```python
from build123d import *

# Parameters (mm, degrees)
EXTRUDE_1_DEPTH     = 80
SKETCH_3_R          = 17.5
EXTRUDE_2_DEPTH     = 10
EXTRUDE_START       = 10
SKETCH_4_R          = 17.5
EXTRUDE_3_DEPTH     = 10
SKETCH_6_R          = 9.5
CUT_EXTRUDE_3_DEPTH = 6
CUT_EXTRUDE_START   = -6
SKETCH_7_R          = 9.5
CUT_EXTRUDE_4_DEPTH = 6
SKETCH_8_R          = 6.5
CUT_EXTRUDE_5_DEPTH = 100
SKETCH_11_R         = 14.5
CUT_EXTRUDE_8_DEPTH = 3
SKETCH_13_R         = 17.5
EXTRUDE_5_DEPTH     = 10


with BuildPart() as part:
    # 草图1 → 凸台-拉伸1 (new body)
    with BuildSketch(Plane.XY):
        Polygon((-20, 18), (-18, 20), (17.735809733, 20), (20, 18), (20, -17.735809733), (17.735809733, -20), (-18, -20), (-20, -18), align=None)
    extrude(amount=EXTRUDE_1_DEPTH)

    # 草图3 → 凸台-拉伸2 (add)
    with BuildSketch(Plane.XY.offset(80)):
        Circle(SKETCH_3_R)
    extrude(amount=EXTRUDE_2_DEPTH)

    # 草图4 → 凸台-拉伸3 (add)
    with BuildSketch(Plane(origin=(0, 0, 0), x_dir=(-1, 0, 0), z_dir=(0, 0, -1)).offset(EXTRUDE_START)):
        with Locations(Location((0, 0, 0), (0, 0, 180))):
            Circle(SKETCH_4_R)
    extrude(amount=-EXTRUDE_3_DEPTH)

    # 草图6 → 切除-拉伸3 (cut)
    with BuildSketch(Plane(origin=(0, 0, -10), x_dir=(-1, 0, 0), z_dir=(0, 0, -1))):
        Circle(SKETCH_6_R)
    extrude(amount=-CUT_EXTRUDE_3_DEPTH, mode=Mode.SUBTRACT)

    # 草图7 → 切除-拉伸4 (cut)
    with BuildSketch(Plane.XY.offset(90).offset(CUT_EXTRUDE_START)):
        with Locations(Location((0, 0, 0), (0, 0, 180))):
            Circle(SKETCH_7_R)
    extrude(amount=CUT_EXTRUDE_4_DEPTH, mode=Mode.SUBTRACT)

    # 草图8 → 切除-拉伸5 (cut)
    with BuildSketch(Plane(origin=(0, 0, -10), x_dir=(-1, 0, 0), z_dir=(0, 0, -1))):
        Circle(SKETCH_8_R)
    extrude(amount=-CUT_EXTRUDE_5_DEPTH, mode=Mode.SUBTRACT)

    # 草图11 → 切除-拉伸8 (cut)
    with BuildSketch(Plane.XY.offset(61.11)):
        Polygon((17.735809733, -20), (-18, -20), (-20, -18), (-20, 18), (-18, 20), (17.735809733, 20), (20, 18), (20, -17.735809733), align=None)
        Circle(SKETCH_11_R, mode=Mode.SUBTRACT)
    extrude(amount=-CUT_EXTRUDE_8_DEPTH, mode=Mode.SUBTRACT)

    # 草图13 → 凸台-拉伸5 (add)
    with BuildSketch(Plane.XY.offset(80)):
        Polygon((-20, 18), (-20, -18), (-18, -20), (17.735809733, -20), (20, -17.735809733), (20, 18), (17.735809733, 20), (-18, 20), align=None)
        with Locations(Location((0, 0, 0), (0, 0, 180))):
            Circle(SKETCH_13_R, mode=Mode.SUBTRACT)
    extrude(amount=EXTRUDE_5_DEPTH)


solid = part.part
```
Input: part model. Units: mm. Frame: model coordinates. A direction names the side the tool comes from. Give positions to 0.01 mm unless a question says otherwise; leave off trailing zeros. Order: outer loops, then holes, each group sorted by start corner. A loop starts at its lowest first (then second) coordinate and runs counter-clockwise, first axis right, second up. Notation, with made-up numbers: M -11.5,74.25 L 20.5,74.25 A13 cw 20.5,83.25 Z; hole C -33.5,-10 d10. An arc over 180 degrees is marked long. Return JSON: item names as keys, results as strings.
1) Line query: L1, parallel to Y at x = 0, z = -7.45; L2, parallel to Z at x = -7, y = 13; L3, parallel to Z at x = 17, y = -16.5. Output: solid intervals per line, ascending. Write a range as [from, to].
Taken from the geometry:
{"L1": "y = [-17.5, -9.5], [9.5, 17.5]", "L2": "z = [-10, 58.11], [61.11, 90]", "L3": "z = [0, 58.11], [61.11, 90]"}
2) Section query C-C on z = 41.5. Output: boundary loops of the cut face in (x, y), and give its area (3 significant figures).
Taken from the geometry:
{"outline": "M -20,-18 L -18,-20 L 17.74,-20 L 20,-17.74 L 20,18 L 17.74,20 L -18,20 L -20,18 Z; hole C 0,0 d13", "area": "1,460 mm2"}
3) Section query D-D on x = -16.5. Output: boundary loops of the cut face in (y, z).
Taken from the geometry:
{"outline": "M -20,0 L -5.83,0 L -5.83,-10 L 5.83,-10 L 5.83,0 L 20,0 L 20,58.11 L -20,58.11 Z; M -20,61.11 L 20,61.11 L 20,90 L -20,90 Z"}
4) Contact query for a flat-ended pin moving along its axis: pin 1 (17 mm diameter, centred on x = 0, y = 0, fed in from +Z). Output: stop coordinate, or through.
Taken from the geometry:
{"pin 1": "stops at z = 84"}
5) Section query A-A on x = 0. Output: boundary loops of the cut face in (y, z).
Taken from the geometry:
{"outline": "M -20,0 L -17.5,0 L -17.5,-10 L -9.5,-10 L -9.5,-4 L -6.5,-4 L -6.5,84 L -9.5,84 L -9.5,90 L -20,90 L -20,61.11 L -14.5,61.11 L -14.5,58.11 L -20,58.11 Z; M 6.5,-4 L 9.5,-4 L 9.5,-10 L 17.5,-10 L 17.5,0 L 20,0 L 20,58.11 L 14.5,58.11 L 14.5,61.11 L 20,61.11 L 20,90 L 9.5,90 L 9.5,84 L 6.5,84 Z"}
6) Mould query, pull axis X, two halves, no side actions, for faces 4 (the face through (5.158, -3.955, 39.384)), 5 (the face through (18.852, -18.884, 75.353)), 6 (the face through (8, 8, -10)). Classes: released by +X, released by -X, zero draft, split by the parting line, or undercut.
Taken from the geometry:
{"face 4": "undercut", "face 5": "released by +X", "face 6": "zero draft"}
7) Access query for faces 1 (the face through (-9, 14, 61.11)), 2 (the face through (-4, -6, -4)), 3 (the face through (0, -20, 29)). Directions: +Z, -Z, +X, -X, +Y, -Y. A direction counts if a zero-diameter tool reaches every point of the face in a straight line with its end or side. Return the directions, or none.
Taken from the geometry:
{"face 1": "none", "face 2": "-Z", "face 3": "+Z, -Z, +X, -X, -Y"}
